Read the model definition and answer for the solid it produces. Units are mm, in the model's axes. Coordinates: 2 decimals unless noted, no trailing zeros. Write each loop counter-clockwise with the first axis right and the second up, starting at its lowest first coordinate (ties: lowest second). Pieces come first, ordered by that corner, then holes. Notation, with made-up numbers: (14.5, -19) -> (29.5, -19) arc R12 ccw to (29.5, 4) -> close; hole circle Ø3 at (22, 12). An arc over 180 degrees is marked (long way). Answer as a JSON object with one key per item and string values. Group by question number.
(1) Find section B-B (y = 15.5). Give the vertices of the cut face in (x, z).
(2) A flat-ended cylindrical pin translates along its axis: P1, Ø1, axis at x = 138, y = -12, coming from the -Z side. Find the tip coordinate at first contact, or state that the pin passes through.
(3) Straight lines are drawn through the part: L1, parallel to X at y = -51, z = 4.1; L2, parallel to X at y = 67, z = 2.15. For each, find the intervals that lie inside material, in ascending order.
(4) Find section A-A (x = -230). Give the vertices of the cut face in (y, z).
from build123d import *

# Parameters (mm, degrees)
F1_DEPTH = 6


with BuildPart() as f1:
    # F0 (on Top) → F1 (new body)
    with BuildSketch(Plane.XY):
        with BuildLine():
            ThreePointArc((275, 170), (270.606602, 180.606602), (260, 185))
            Line((260, 185), (-260, 185))
            ThreePointArc((-260, 185), (-270.606602, 180.606602), (-275, 170))
            Line((-275, 170), (-275, -170))
            ThreePointArc((-275, -170), (-270.606602, -180.606602), (-260, -185))
            Line((-260, -185), (260, -185))
            ThreePointArc((260, -185), (270.606602, -180.606602), (275, -170))
            Line((275, -170), (275, 170))
        make_face()
        with BuildLine():
            ThreePointArc((-215.015495, 65.681628), (-215, 65.001779), (-215.015334, 64.321926))
            Line((-215.015334, 64.321926), (-215, -64.998221))
            ThreePointArc((-215, -64.998221), (-229.443822, -79.989685), (-244.958887, -66.109818))
            ThreePointArc((-244.958887, -66.109818), (-245, -65), (-244.958887, -63.890182))
            Line((-244.958887, -63.890182), (-244.958887, 63.890182))
            ThreePointArc((-244.958887, 63.890182), (-245, 65), (-244.958887, 66.109818))
            ThreePointArc((-244.958887, 66.109818), (-229.785522, 79.998467), (-215.015495, 65.681628))
        make_face(mode=Mode.SUBTRACT)
    extrude(amount=F1_DEPTH)


solid = f1.part
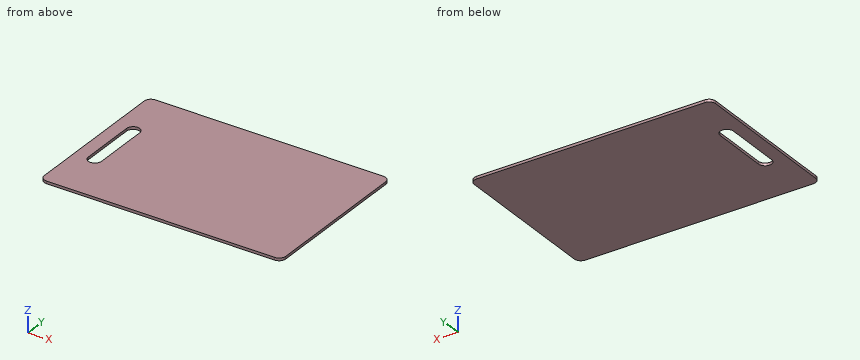
Results below:
{
 "1": {"outline": "(-275, 0) -> (-244.96, 0) -> (-244.96, 6) -> (-275, 6) -> close; (-215.01, 0) -> (275, 0) -> (275, 6) -> (-215.01, 6) -> close"},
 "2": {"P1": "stops at z = 0"},
 "3": {"L1": "x = -275 to -244.96, -215 to 275", "L2": "x = -275 to -244.87, -215.13 to 275"},
 "4": {"outline": "(-185, 0) -> (-80, 0) -> (-80, 6) -> (-185, 6) -> close; (80, 0) -> (185, 0) -> (185, 6) -> (80, 6) -> close"}
}
